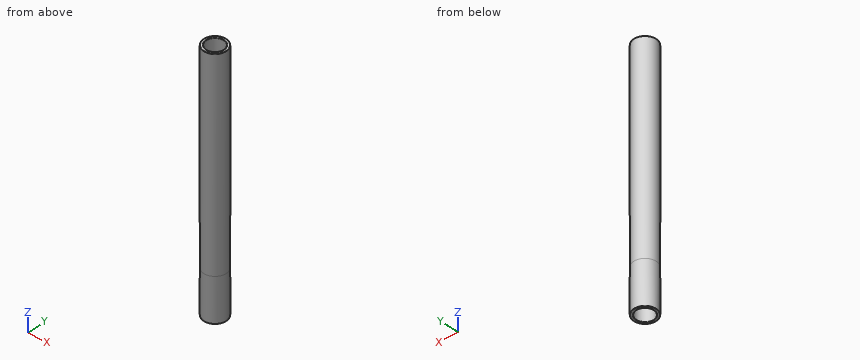
Autodesk Inventor part; units mm, degrees
ref_plane "YZ Plane" through (0, 0, 0) normal (1, 0, 0) x (0, 1, 0)
ref_plane "XZ Plane" through (0, 0, 0) normal (0, 1, 0) x (-1, 0, 0)
ref_plane "XY Plane" through (0, 0, 0) normal (0, 0, 1) x (1, 0, 0)
sketch "草圖1" plane through (0, 0, 0) normal (0, 1, 0) x (-1, 0, 0)
  line L0 (0, 0) -> (0, -99)
  line L1 (0, -99) -> (4.5, -99)
  line L2 (4.5, -99) -> (4.5, 0)
  line L3 (4.5, 0) -> (0, 0)
  line L4 (0, -99) -> (0, -81.5)
  line L5 (0, -81.5) -> (4.5, -81.5)
  dimension "d0" = 99
  dimension "d1" = 4.5
  dimension "d2" = 90
  dimension "d4" = 17.5
revolve "迴轉3" add sketch "草圖1" angle 360 about axis through (-4.5, 0, -99) along (0, 0, 1) contours L3 L2 L5 L0
sketch "草圖3" plane through (-4.5, 0, -81.5) normal (0, 0, -1) x (-1, 0, 0)
  point P0 (-4.5, 0)
  point P1 (-0.0147, -0.0564)
hole "孔2" at (-4.4853, -0.0564, -81.5) direction (0, 0, 1) diameter 5 depth 66.5 tip angle 118
sketch "草圖4" plane through (-4.5, 0, 0) normal (0, 0, 1) x (1, 0, 0)
  point P0 (4.5, 0)
  point P1 (-0.0009, 0.0083)
hole "孔3" at (-4.5009, 0.0083, 0) direction (0, 0, -1) diameter 7 depth 15 tip angle 118
sketch "草圖5" plane through (-4.5, 0, -81.5) normal (0, 0, -1) x (-1, 0, 0)
  circle A0 centre (0, 0) radius 4.5
  point P0 (-4.5, 0)
extrude "擠出1" add sketch "草圖5" along normal blind 17.5
sketch "草圖6" plane through (-4.5, 0, -99) normal (0, 0, -1) x (-1, 0, 0)
  point P0 (-4.5, 0)
  point P1 (-0.0069, -0.0273)
hole "孔4" at (-4.4931, -0.0273, -99) direction (0, 0, 1) diameter 7 depth 17.5 tip angle 118
fillet "圓角1" radius 0.15 1 edges at (-9, 0, 0)
fillet "圓角2" radius 0.15 3 edges at (-4.5009, 3.5083, 0) (-4.4931, -3.5273, -99) (0, 0, -99)
properties part number "筆桿"
Part model, mm, in its own coordinate system. Round coordinates to 2 decimals unless told otherwise and drop trailing zeros. Loops run counter-clockwise (first coordinate to the right, second up) from the corner with the lowest first, then second, coordinate; pieces in that order, holes last. Notation, with made-up numbers: (23, 36.25) -> (35, 36.25) arc R12 cw to (35, 49.25) -> close; hole circle Ø11 at (32.5, 19.25). An arc over 180 degrees is marked (long way). Use CSV: the item, a comma, the result in double quotes. Start each with the question number.
1) Cut at A-A, the plane z = -24. Write the cut outline in (x, y).
2) Cut at B-B, the plane z = -8.5. Write the cut outline in (x, y), plus the area to 3 significant figures.
3) Wall check: L1, parallel to Y at x = -4.75, z = -18.5; L2, parallel to Y at x = -5.5, z = -24; L3, parallel to X at y = -1.75, z = -6. Give the ranges that are in metal, low to high. Write a range as [from, to].
Determined:
1,outline,"circle Ø9 at (-4.5, 0); hole circle Ø5 at (-4.49, -0.06)"
2,outline,"circle Ø9 at (-4.5, 0); hole circle Ø7 at (-4.5, 0.01)"
2,area,"25.1 mm2"
3,L1,"y = [-4.49, -2.54], [2.43, 4.49]"
3,L2,"y = [-4.39, -2.34], [2.23, 4.39]"
3,L3,"x = [-8.65, -7.53], [-1.47, -0.35]"
